```python
from build123d import *

# Parameters (mm, degrees)
SKETCH1_W           = 81.2
SKETCH1_H           = 81.2
BOSS_EXTRUDE1_DEPTH = 1
SKETCH1_4_W         = 14
SKETCH1_4_H         = 6.5
BOSS_EXTRUDE3_DEPTH = 4
CUT_EXTRUDE1_START  = 1
SKETCH1_5_W         = 10
SKETCH1_5_H         = 3
CUT_EXTRUDE1_DEPTH  = 2
CIRPATTERN2_COUNT   = 4


with BuildPart() as part:
    # Sketch1 → Boss-Extrude1 (new body)
    with BuildSketch(Plane(origin=(0, 0, 0), x_dir=(1, 0, 0), z_dir=(0, 1, 0))):
        with Locations((4.005258085, 4.818334453)):
            Rectangle(SKETCH1_W, SKETCH1_H)
    extrude(amount=-BOSS_EXTRUDE1_DEPTH)

    # Sketch1<4> → Boss-Extrude3 (add)
    with BuildSketch(Plane(origin=(0, 0, 0), x_dir=(1, 0, 0), z_dir=(0, 1, 0))):
        with Locations((4.005258085, 40.168334453)):
            Rectangle(SKETCH1_4_W, SKETCH1_4_H)
    boss_extrude3 = extrude(amount=BOSS_EXTRUDE3_DEPTH)

    # Sketch1<5> → Cut-Extrude1 (cut)
    with BuildSketch(Plane(origin=(0, 0, 0), x_dir=(1, 0, 0), z_dir=(0, 1, 0)).offset(CUT_EXTRUDE1_START)):
        with Locations((4.005258085, 39.918334453)):
            Rectangle(SKETCH1_5_W, SKETCH1_5_H)
    cut_extrude1 = extrude(amount=CUT_EXTRUDE1_DEPTH, mode=Mode.SUBTRACT)

    # CirPattern2: Boss-Extrude3, Cut-Extrude1 ×4 about axis
    cirpattern2_axis = Axis((4.005258085, 0, -4.818334453), (0, 1, 0))
    add([boss_extrude3.rotate(cirpattern2_axis, i * 360 / CIRPATTERN2_COUNT) for i in range(1, CIRPATTERN2_COUNT)])
    add([cut_extrude1.rotate(cirpattern2_axis, i * 360 / CIRPATTERN2_COUNT) for i in range(1, CIRPATTERN2_COUNT)], mode=Mode.SUBTRACT)


solid = part.part
```
Input: part model. Units: mm. Frame: model coordinates. A direction names the side the tool comes from. Coordinates: 2 decimals unless noted, no trailing zeros. Loops run counter-clockwise (first coordinate to the right, second up) from the corner with the lowest first, then second, coordinate; pieces in that order, holes last. Notation, with made-up numbers: M 16,11.5 L 45,11.5 A22 cw 45,35.5 Z; hole C 25,9.25 d8. An arc over 180 degrees is marked long. One line per item, written item: value.
(1) Section A-A (y = 1.95). Give the number of separate pieces and of enclosed holes in the cut face, and give its area (3 significant figures).
Filled in:
separate pieces: 4
enclosed holes: 4
area: 244 mm^2
(2) Section B-B (z = -1). Output: boundary loops of the cut face in (x, y), and give its area (3 significant figures).
Filled in:
outline: M -36.59,-1 L 44.61,-1 L 44.61,0 L 42.61,0 L 42.61,4 L 36.11,4 L 36.11,0 L -28.09,0 L -28.09,4 L -34.59,4 L -34.59,0 L -36.59,0 Z; hole M -32.59,1 L -29.59,1 L -29.59,3 L -32.59,3 Z; hole M 37.61,1 L 40.61,1 L 40.61,3 L 37.61,3 Z
area: 121 mm^2
(3) Section D-D (x = 1). Output: boundary loops of the cut face in (y, z), and give its area (3 significant figures).
Filled in:
outline: M -1,-45.42 L 0,-45.42 L 0,-43.42 L 4,-43.42 L 4,-36.92 L 0,-36.92 L 0,27.28 L 4,27.28 L 4,33.78 L 0,33.78 L 0,35.78 L -1,35.78 Z; hole M 1,-41.42 L 3,-41.42 L 3,-38.42 L 1,-38.42 Z; hole M 1,28.78 L 3,28.78 L 3,31.78 L 1,31.78 Z
area: 121 mm^2
(4) Line query: line 1 along Z through (x, y) = (-0.5, 2.7); line 2 along Y through (x, z) = (-31, 31.5); line 3 along Z through (x, y) = (41, 0.95). Output: solid intervals per line, ascending. Write a range as from..to.
Filled in:
line 1: -43.42..-41.42, -38.42..-36.92, 27.28..28.78, 31.78..33.78
line 2: -1..0
line 3: -11.82..2.18
(5) Pin query (flat end, axial travel): pin 1 (0.6 mm diameter, centred on x = 3, y = 2.5, fed in from -Z); pin 2 (1.2 mm diameter, centred on y = 3, z = -3, fed in from -X); pin 3 (1 mm diameter, centred on x = 39.5, y = 2, fed in from -Z); pin 4 (5 mm diameter, centred on x = 6, z = 26, fed in from +Y). Return the tip coordinate at first contact, or that it passes through.
Filled in:
pin 1: z = -43.42
pin 2: x = -34.59
pin 3: z = -11.82
pin 4: y = 4
(6) Section C-C (x = 39.5). Output: boundary loops of the cut face in (y, z), and give its area (3 significant figures).
Filled in:
outline: M -1,-45.42 L 0,-45.42 L 0,-11.82 L 4,-11.82 L 4,2.18 L 0,2.18 L 0,35.78 L -1,35.78 Z; hole M 1,-9.82 L 3,-9.82 L 3,0.18 L 1,0.18 Z
area: 117 mm^2
(7) Pull-direction query (Z, two-part tool) for faces 1 (the flat face through (39, 2, -11.818)), 2 (the flat face through (42.605, 2, -5)), 3 (the flat face through (4, 2, 31.782)); classes: +Z half, -Z half, draft (parallel to the pull), parting line (faces both ways), or undercut.
Filled in:
face 1: -Z half
face 2: draft
face 3: undercut
(8) Reachability of faces 4 (the flat face through (-0.995, 2, -40)), 5 (the flat face through (36.105, 2, -5)), 6 (the flat face through (4, 2, -36.918)), 7 (the flat face through (-2.995, 2, 30)), 8 (the flat face through (11.005, 2, -40)) from +Z, -Z, +X, -X, +Y, -Y: full face, straight path, thin tool, end or side. Return the list, or none.
Filled in:
face 4: none
face 5: +Z, -Z, +Y
face 6: +X, -X, +Y
face 7: +Z, -Z, -X, +Y
face 8: +Z, -Z, +X, +Y
